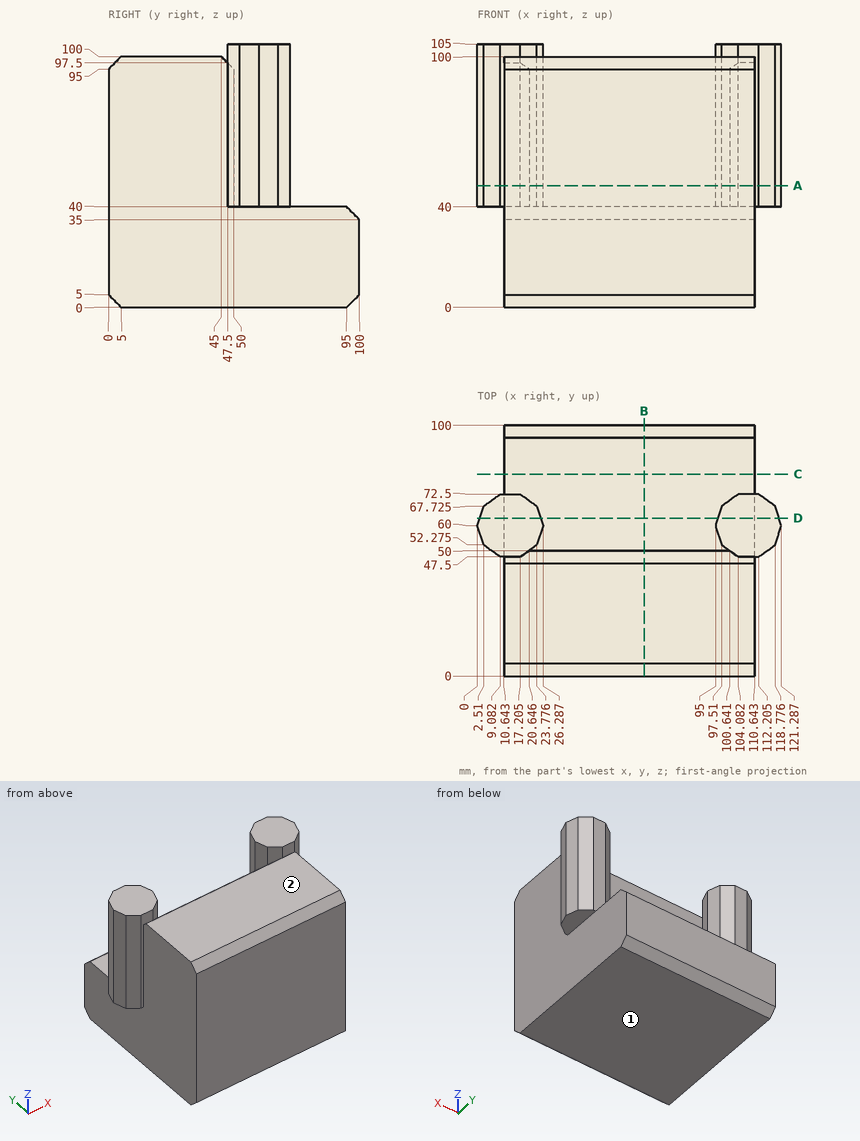
Print and shaded views of the part. All mm, measured from the part's lowest x, y and z. A direction names the side the tool comes from. Give positions to 0.01 mm unless a question says otherwise; leave off trailing zeros. Loops run counter-clockwise (first coordinate to the right, second up) from the corner with the lowest first, then second, coordinate; pieces in that order, holes last. Notation, with made-up numbers: (49.25, 30.5) - (73.25, 30.5) arc R13 ccw to (73.25, 41.5) - close; hole circle Ø10 at (63.5, 4.25). An arc over 180 degrees is marked (long way). One line per item, written item: value. Start each with the question number.
1. Slice it at D-D (y = 63). List the corners of the cut face in (x, z) (1 decimal), plus the area to 3 significant figures.
2. Which spindle directions (+Z, -Z, +X, -X, +Y, -Y) get a long thin tool onto all of the face, cutting with end or side? Do the marked faces 1 and 2. Say none if no direction does.
3. Probe L1, parallel to X at y = 42, z = 89.5; L2, parallel to Y at x = 105.5, z = 78.5; L3, parallel to Y at x = 42, z = 92. List the from-to ranges inside material, lowest first. Write a range as from..to.
4. Slice it at C-C (y = 80.5). List the corners of the cut face in (x, z).
5. Slice it at B-B (x = 66.5). List the corners of the cut face in (y, z), plus the area to 3 significant figures.
6. Pin check, flat tips, straight feed: pin 1 (6.5 mm diameter, centred on x = 11.5, z = 60, fed in from +Y); pin 2 (3 mm diameter, centred on x = 116, y = 57.5, fed in from -Z); pin 3 (22.5 mm diameter, centred on x = 80, y = 74, fed in from +Z). Stop position of each tip, or through.
7. Slice it at A-A (z = 48.5). List the corners of the cut face in (x, y) (1 decimal), plus the area to 3 significant figures.
Solution:
1. outline: (1, 40) - (10.6, 40) - (10.6, 0) - (110.6, 0) - (110.6, 40) - (120.3, 40) - (120.3, 105) - (96, 105) - (96, 40) - (25.3, 40) - (25.3, 105) - (1, 105) - close
1. area: 7,160 mm^2
2. face 1: -Z, +X, -X, +Y, -Y
2. face 2: +Z, +X, -X, -Y
3. L1: x = 10.64..110.64
3. L2: y = 0..72.5
3. L3: y = 0..50
4. outline: (10.64, 0) - (110.64, 0) - (110.64, 40) - (10.64, 40) - close
5. outline: (0, 5) - (5, 0) - (95, 0) - (100, 5) - (100, 35) - (95, 40) - (50, 40) - (50, 95) - (45, 100) - (5, 100) - (0, 95) - close
5. area: 6,940 mm^2
6. pin 1: stops at y = 72.5
6. pin 2: stops at z = 40
6. pin 3: stops at z = 40
7. outline: (0, 60) - (2.5, 52.3) - (9.1, 47.5) - (10.6, 47.5) - (10.6, 0) - (110.6, 0) - (110.6, 47.5) - (112.2, 47.5) - (118.8, 52.3) - (121.3, 60) - (118.8, 67.7) - (112.2, 72.5) - (104.1, 72.5) - (97.5, 67.7) - (95, 60) - (97.5, 52.3) - (100.6, 50) - (20.6, 50) - (23.8, 52.3) - (26.3, 60) - (23.8, 67.7) - (17.2, 72.5) - (9.1, 72.5) - (2.5, 67.7) - close
7. area: 5,970 mm^2
